```python
from build123d import *

# Parameters (mm, degrees)
BOSS_EXTRUDE2_DEPTH = 13
CHAMFER2_SIZE       = 3


with BuildPart() as part:
    # Sketch1 → Boss-Extrude2 (new body)
    with BuildSketch(Plane(origin=(0, 0, 0), x_dir=(1, 0, 0), z_dir=(0, 1, 0))):
        with BuildLine():
            Line((10, 0), (548, 0))
            ThreePointArc((548, 0), (555.071067812, 2.928932188), (558, 10))
            Line((558, 10), (558, 448))
            ThreePointArc((558, 448), (555.071067812, 455.071067812), (548, 458))
            Line((548, 458), (489, 458))
            ThreePointArc((489, 458), (481.928932188, 460.928932188), (479, 468))
            Line((479, 468), (479, 790))
            ThreePointArc((479, 790), (476.071067812, 797.071067812), (469, 800))
            Line((469, 800), (89, 800))
            ThreePointArc((89, 800), (81.928932188, 797.071067812), (79, 790))
            Line((79, 790), (79, 468))
            ThreePointArc((79, 468), (76.071067812, 460.928932188), (69, 458))
            Line((69, 458), (10, 458))
            ThreePointArc((10, 458), (2.928932188, 455.071067812), (0, 448))
            Line((0, 448), (0, 10))
            ThreePointArc((0, 10), (2.928932188, 2.928932188), (10, 0))
        make_face()
    extrude(amount=BOSS_EXTRUDE2_DEPTH)

    # Chamfer2
    chamfer2_edges = [part.edges().sort_by_distance(p)[0] for p in [
        (81.928932188, 13, -797.071067812),
        (79, 13, -629),
        (76.071067812, 13, -460.928932188),
        (39.5, 13, -458),
        (2.928932188, 13, -455.071067812),
        (0, 13, -229),
        (2.928932188, 13, -2.928932188),
        (279, 13, 0),
        (555.071067812, 13, -2.928932188),
        (558, 13, -229),
        (476.071067812, 13, -797.071067812),
        (555.071067812, 13, -455.071067812),
        (518.5, 13, -458),
        (481.928932188, 13, -460.928932188),
        (479, 13, -629),
        (279, 13, -800),
    ]]
    chamfer(chamfer2_edges, length=CHAMFER2_SIZE)


solid = part.part
```
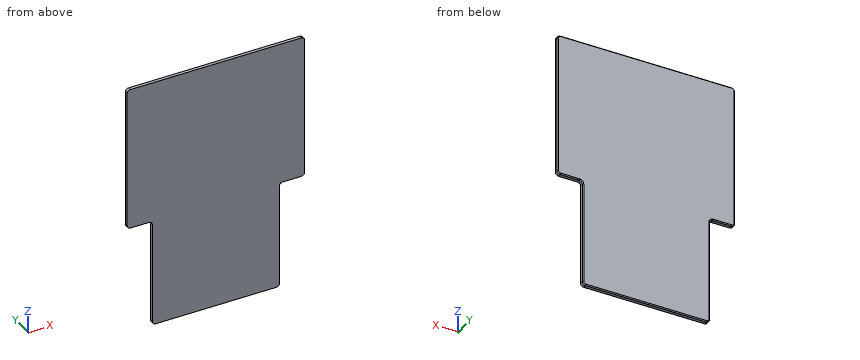
Model file for the job. Use its own axes, mm. Coordinates: 2 decimals unless noted, no trailing zeros. Write each loop counter-clockwise with the first axis right and the second up, starting at its lowest first coordinate (ties: lowest second). Pieces come first, ordered by that corner, then holes. Notation, with made-up numbers: (-9.75, 46) - (36.25, 46) arc R33 ccw to (36.25, 74) - close; hole circle Ø5 at (2.25, -32.5). An arc over 180 degrees is marked (long way). One line per question, with ' | ' between items. Start each with the question number.
Q1. Cut at B-B, the plane z = -742.5. List the corners of the cut face in (x, y).
Q2. Cut at C-C, the plane x = 513.5. List the corners of the cut face in (y, z).
Q3. Drill centre lines: line 1 (Z direction, x = 490, y = 2); line 2 (X direction, y = 7.5, z = -448.5); line 3 (Z direction, x = 82, y = 1.5). Where is each one in solid material? Low to high. Write a range as [from, to].
Q4. Cut at A-A, the plane y = 4. List the corners of the cut face in (x, z).
Q5. Pin check, flat tips, straight feed: pin 1 (3 mm diameter, centred on x = 518, y = 4.5, fed in from -Z); pin 2 (3 mm diameter, centred on y = 3.5, z = -605.5, fed in from +X). Stop position of each tip, or through.
Answer below:
1) outline: (79, 0) - (479, 0) - (479, 10) - (476, 13) - (82, 13) - (79, 10) - close
2) outline: (0, -458) - (10, -458) - (13, -455) - (13, -3) - (10, 0) - (0, 0) - close
3) line 1: [-458, 0] | line 2: [0.01, 557.99] | line 3: [-797.14, 0]
4) outline: (0, -448) arc R10 ccw to (10, -458) - (69, -458) arc R10 cw to (79, -468) - (79, -790) arc R10 ccw to (89, -800) - (469, -800) arc R10 ccw to (479, -790) - (479, -468) arc R10 cw to (489, -458) - (548, -458) arc R10 ccw to (558, -448) - (558, -10) arc R10 ccw to (548, 0) - (10, 0) arc R10 ccw to (0, -10) - close
5) pin 1: z = -458 | pin 2: x = 479
